Verification items for the finished model (mm, model axes). Face numbers are marked on the shaded views. A direction names the side the tool comes from. Give positions to 0.01 mm unless a question says otherwise; leave off trailing zeros. Loops run counter-clockwise (first coordinate to the right, second up) from the corner with the lowest first, then second, coordinate; pieces in that order, holes last. Notation, with made-up numbers: (80, 43) - (97, 43) arc R24 cw to (97, 65) - close; hole circle Ø6 at (-11, -26.75). An arc over 180 degrees is marked (long way). Answer in a Markdown table with one row per item.
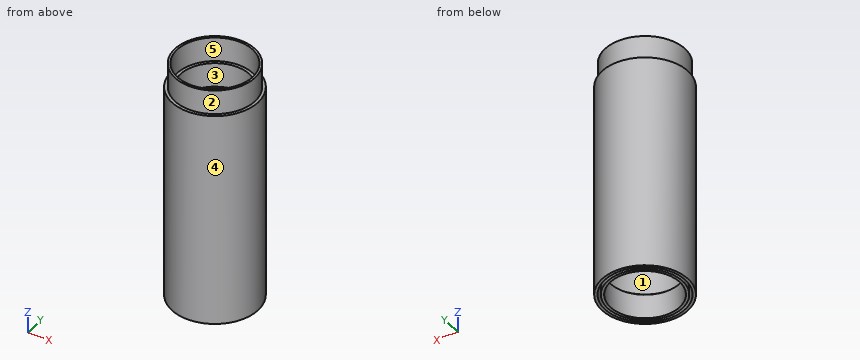
```python
from build123d import *

# Parameters (mm, degrees)
F0_W   = 1.5
F0_H   = 13
F0_W_2 = 1.2


with BuildPart() as f1:
    # F0 (on Front) → F1 (revolve)
    with BuildSketch(Plane.XZ):
        with BuildLine():
            Line((20, 87.5), (20, 44.5))
            Line((20, 44.5), (23, 44.5))
            Line((23, 44.5), (23, 102))
            Line((23, 102), (21.35, 102))
            Line((21.35, 102), (20.15, 102))
            Line((20.15, 102), (18.5, 102))
            Line((18.5, 102), (18.5, 89))
            ThreePointArc((18.5, 89), (19.56066, 88.56066), (20, 87.5))
        make_face()
        Polygon((20, 1.5), (20, 0), (21.5, 0), (23, 0), (23, 44.5), (20, 44.5), align=None)
        with Locations((22.25, -6.5)):
            Rectangle(F0_W, F0_H)
        with Locations((19.25, -6.5)):
            Rectangle(F0_W, F0_H)
        with BuildLine():
            ThreePointArc((20, 1.5), (19.56066, 0.43934), (18.5, 0))
            Line((18.5, 0), (20, 0))
            Line((20, 0), (20, 1.5))
        make_face()
        with Locations((20.75, 108.5)):
            Rectangle(F0_W_2, F0_H)
    revolve(axis=Axis((0, 0, 51), (0, 0, 1)))


solid = f1.part
```
Q1. Sectioned sample at D-D (z = -5). Record the cut outline in (x, y).
Completed:
| item | result |
|---|---|
| outline | circle Ø46 at (0, 0); circle Ø40 at (0, 0); hole circle Ø43 at (0, 0); hole circle Ø37 at (0, 0) |
Q2. Tool access check on the marked faces 1, 2 and 3. Record the directions out of +Z, -Z, +X, -X, +Y, -Y that give a thin tool (end or side, any length) a straight path to the whole face; none if there is none.
Completed:
| item | result |
|---|---|
| face 1 | none |
| face 2 | +Z |
| face 3 | +Z, -Z |
Q3. Draft check along Y on the marked faces 4 and 5. Enter one of: +Y half, -Y half, draft (parallel to the pull), parting line (faces both ways), or undercut.
Completed:
| item | result |
|---|---|
| face 4 | parting line |
| face 5 | undercut |
Q4. Go/stop test with flat-tipped pins: P1, Ø1, axis at y = 10.5, z = 64, coming from the -X side; P2, Ø10, axis at x = 14.5, z = 5.5, coming from the +Y side; P3, Ø1, axis at x = 12, z = 50, coming from the -Y side. Record where each tip stops, or that it passes through.
Completed:
| item | result |
|---|---|
| P1 | x = -20.71 |
| P2 | y = 20.95 |
| P3 | y = -19.92 |
Q5. Thickness scan on line 1 (Y direction, x = 0, z = -10); line 2 (Y direction, x = 0, z = 29); line 3 (Y direction, x = 0, z = 97.5). Record the ranges inside material, lowest first.
Completed:
| item | result |
|---|---|
| line 1 | -23 to -21.5, -20 to -18.5, 18.5 to 20, 21.5 to 23 |
| line 2 | -23 to -20, 20 to 23 |
| line 3 | -23 to -18.5, 18.5 to 23 |
Q6. Sectioned sample at C-C (z = 85). Record the cut outline in (x, y), and give its area (3 significant figures).
Completed:
| item | result |
|---|---|
| outline | circle Ø46 at (0, 0); hole circle Ø40 at (0, 0) |
| area | 405 mm^2 |
